```python
from build123d import *

# Parameters (mm, degrees)
BOSS_EXTRUDE1_DEPTH = 4.5
BOSS_EXTRUDE2_DEPTH = 3.8
BOSS_EXTRUDE3_DEPTH = 8.1
SKETCH5_W           = 103.25
SKETCH5_H           = 49.520314098
BOSS_EXTRUDE4_DEPTH = 2
FILLET1_R           = 7
SKETCH6_W           = 74.836382047
SKETCH6_H           = 26.769621583
CUT_EXTRUDE1_DEPTH  = 0.42


with BuildPart() as part:
    # Sketch1 → Boss-Extrude1 (new body)
    with BuildSketch(Plane(origin=(0, 0, 0), x_dir=(1, 0, 0), z_dir=(0, 1, 0))):
        with BuildLine():
            Line((7.25, 0), (7.25, -35))
            ThreePointArc((7.25, -35), (0, -42.25), (-7.25, -35))
            Line((-7.25, -35), (-7.25, 0))
            ThreePointArc((-7.25, 0), (0, 7.25), (7.25, 0))
        make_face()
    extrude(amount=BOSS_EXTRUDE1_DEPTH)

    # Sketch3 → Boss-Extrude2 (add)
    with BuildSketch(Plane(origin=(0, 4.5, 0), x_dir=(1, 0, 0), z_dir=(0, 1, 0))):
        with BuildLine():
            Line((-2.622571491, -0.457666807), (-2.622571491, -0.011296081))
            Line((-2.622571491, -0.011296081), (2.763792269, -0.011296081))
            Line((2.763792269, -0.011296081), (2.763792269, -0.457666807))
            ThreePointArc((2.763792269, -0.457666807), (2.791332039, -0.235236185), (2.800532634, -0.011296081))
            ThreePointArc((2.800532634, -0.011296081), (-0.153329714, 2.709425568), (-2.622571491, -0.457666807))
        make_face()
        with BuildLine():
            Line((2.763792269, -0.011296081), (-2.622571491, -0.011296081))
            Line((-2.622571491, -0.011296081), (-2.622571491, -0.457666807))
            ThreePointArc((-2.622571491, -0.457666807), (0.070610389, -2.741218326), (2.763792269, -0.457666807))
            Line((2.763792269, -0.457666807), (2.763792269, -0.011296081))
        make_face()
        with BuildLine():
            ThreePointArc((2.763792269, -0.457666807), (0.070610389, -2.741218326), (-2.622571491, -0.457666807))
            Line((-2.622571491, -0.457666807), (-2.622571491, -35.011296081))
            ThreePointArc((-2.622571491, -35.011296081), (0.070610389, -32.318114201), (2.763792269, -35.011296081))
            Line((2.763792269, -35.011296081), (2.763792269, -0.457666807))
        make_face()
        with BuildLine():
            ThreePointArc((2.763792269, -35.011296081), (0.070610389, -32.318114201), (-2.622571491, -35.011296081))
            Line((-2.622571491, -35.011296081), (2.763792269, -35.011296081))
        make_face()
        with BuildLine():
            Line((2.763792269, -35.011296081), (-2.622571491, -35.011296081))
            ThreePointArc((-2.622571491, -35.011296081), (0.070610389, -37.704477961), (2.763792269, -35.011296081))
        make_face()
    extrude(amount=BOSS_EXTRUDE2_DEPTH)

    # Sketch4 → Boss-Extrude3 (add)
    with BuildSketch(Plane(origin=(0, 8.3, 0), x_dir=(1, 0, 0), z_dir=(0, 1, 0))):
        with BuildLine():
            Line((7.25308141, 0.014627933), (7.323691799, -34.996668148))
            ThreePointArc((7.323691799, -34.996668148), (0.085238322, -42.264377491), (-7.182471021, -35.025924014))
            Line((-7.182471021, -35.025924014), (-7.25308141, -0.014627933))
            ThreePointArc((-7.25308141, -0.014627933), (-0.014627933, 7.25308141), (7.25308141, 0.014627933))
        make_face()
    extrude(amount=BOSS_EXTRUDE3_DEPTH)

    # Sketch5 → Boss-Extrude4 (add)
    with BuildSketch(Plane(origin=(0, 16.4, 0), x_dir=(1, 0, 0), z_dir=(0, 1, 0))):
        with Locations((44.371903839, -17.507075639)):
            Rectangle(SKETCH5_W, SKETCH5_H)
    extrude(amount=BOSS_EXTRUDE4_DEPTH)

    # Fillet1
    fillet1_edges = [part.edges().sort_by_distance(p)[0] for p in [
        (95.996903839, 17.4, 42.267232688),
        (95.996903839, 17.4, -7.25308141),
        (-7.253096161, 17.4, -7.25308141),
        (-7.253096161, 17.4, 42.267232688),
    ]]
    fillet(fillet1_edges, radius=FILLET1_R)

    # Sketch6 → Cut-Extrude1 (cut)
    with BuildSketch(Plane(origin=(95.996903839, 0, 0), x_dir=(0, 0, -1), z_dir=(1, 0, 0))):
        with Locations((-22.928368507, 17.221399119)):
            Rectangle(SKETCH6_W, SKETCH6_H)
    extrude(amount=-CUT_EXTRUDE1_DEPTH, mode=Mode.SUBTRACT)


solid = part.part
```
Read the model definition and answer for the solid it produces. Units are mm, in the model's axes. A direction names the side the tool comes from. Round coordinates to 2 decimals unless told otherwise and drop trailing zeros. Write each loop counter-clockwise with the first axis right and the second up, starting at its lowest first coordinate (ties: lowest second). Pieces come first, ordered by that corner, then holes. Notation, with made-up numbers: (38.5, 69) - (85.5, 69) arc R33 ccw to (85.5, 99) - close; hole circle Ø8 at (0, 2). An arc over 180 degrees is marked (long way). Use CSV: the item, a comma, the result in double quotes.
Q1. Each of these flat-tipped pins is pushed along its axis until it touches: pin 1 Ø2 at (y, z) = (2, 13.5) entering from -X; pin 2 Ø3.5 at (y, z) = (1.5, 24) entering from +X; pin 3 Ø5 at (x, z) = (11, 0) entering from -Y. Where does it stop, or does it pass through?
Values:
pin 1,"stops at x = -7.25"
pin 2,"stops at x = 7.25"
pin 3,"stops at y = 16.4"
Q2. A tool of negligible diameter and unlimited length cuts with its end or side. For faces 4 (the flat face through (44, 17, 42.267)), 5 (the cylindrical face through (0.16, 2.22, 42.25)), 6 (the cylindrical face through (-0.16, 2.22, -7.25)), from which of +Z, -Z, +X, -X, +Y, -Y can it reach the whole face along a straight path? Write none if from no direction.
Values:
face 4,"+Z, +X, -X, +Y, -Y"
face 5,"+Z, -Y"
face 6,"-Z, -Y"
Q3. Straight lines are drawn through the part: line 1 along Y through (x, z) = (6, 32); line 2 along X through (y, z) = (7.25, 27); line 3 along Y through (x, z) = (90, -4.5). For each, find the intervals that lie inside material, in ascending order.
Values:
line 1,"y = 0 to 4.5, 8.3 to 18.4"
line 2,"x = -2.62 to 2.76"
line 3,"y = 16.4 to 18.4"
Q4. Determine the mould class of faces 1 (the flat face through (-3, 4.5, 17)), 2 (the cylindrical face through (92.965, 17.414, -6.02)), 3 (the flat face through (0, 0, 17)) for opening direction Y: +Y half, -Y half, draft (parallel to the pull), parting line (faces both ways), or undercut.
Values:
face 1,"undercut"
face 2,"draft"
face 3,"-Y half"
Q5. Find section B-B, the plane y = 10. Write down the section's boundary in (x, z), then the cut area to 3 significant figures.
Values:
outline,"(-7.25, 0.01) arc R7.25 ccw to (7.25, -0.01) - (7.32, 35) arc R7.25 ccw to (-7.18, 35.03) - close"
area,"673 mm²"
Q6. Find section C-C, the plane x = 45. Write down the section's boundary in (y, z).
Values:
outline,"(16.4, -7.25) - (18.4, -7.25) - (18.4, 42.27) - (16.4, 42.27) - close"
